For this review, use the dimensioned drawing (mm, ordinates from the lowest corner) and the shaded views. Round coordinates to 2 decimals unless told otherwise and drop trailing zeros. Loops run counter-clockwise (first coordinate to the right, second up) from the corner with the lowest first, then second, coordinate; pieces in that order, holes last. Notation, with made-up numbers: M 62.5,42.25 L 75.5,42.25 A13 cw 75.5,57.25 Z; hole C 10,38.5 d6. An arc over 180 degrees is marked long. Use a Markdown table: item, result. Add a question column.
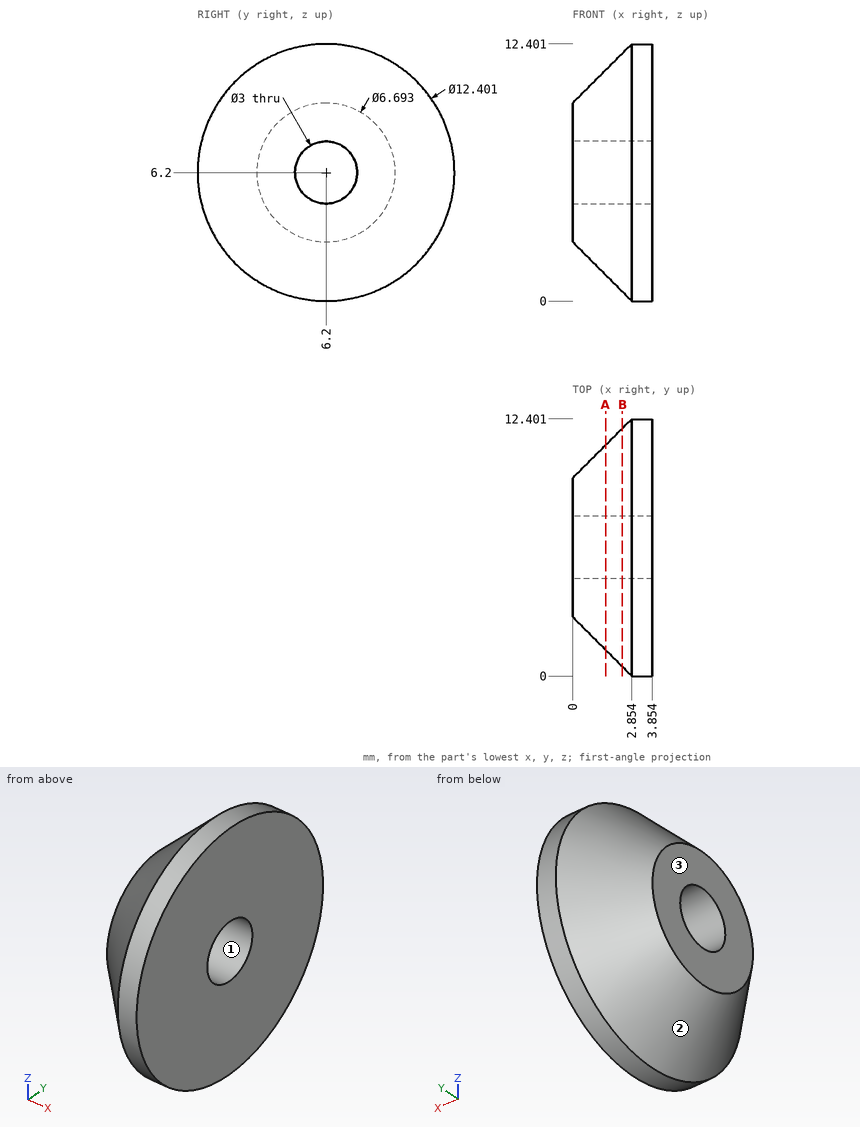
(1) Consider section B-B, the plane x = 2.4. Give the boundary of the cut face in (y, z).
(2) Draft analysis for pull direction Z (two halves, no side actions). For the marked faces 1, 2 and 3, state which applies: released by +Z, released by -Z, zero draft, split by the parting line, or undercut.
(3) To check wall thickness, follow probe 1 along Y at (x, z) = (1.45, 6.5) (1 decimal); probe 2 along Z at (x, y) = (1.7, 6.75) (1 decimal); probe 3 along Y at (x, z) = (3, 5) (1 decimal). State the ranges of each line that lie inside material, in increasing order.
(4) Consider section A-A, the plane x = 1.6. Give the boundary of the cut face in (y, z), then the cut area to 3 significant figures.
(5) Insertion check: pin 1 Ø1 at (x, z) = (1, 7.5) entering from -Y (1 decimal); pin 2 Ø2 at (x, z) = (1, 2) entering from -Y; pin 3 Ø1 at (x, y) = (1, 2.5) entering from +Z (1 decimal). Each pin has a flat end and moves straight along its axis. Give the tip position at first contact, or say it passes through.
Found:
| question | item | result |
|---|---|---|
| 1 | outline | C 6.2,6.2 d11.49; hole C 6.2,6.2 d3 |
| 2 | face 1 | undercut |
| 2 | face 2 | split by the parting line |
| 2 | face 3 | zero draft |
| 3 | probe 1 | y = 1.4 to 4.7, 7.7 to 11 |
| 3 | probe 2 | z = 1.2 to 4.8, 7.6 to 11.2 |
| 3 | probe 3 | y = 0.1 to 5.3, 7.1 to 12.3 |
| 4 | outline | C 6.2,6.2 d9.89; hole C 6.2,6.2 d3 |
| 4 | area | 69.8 mm^2 |
| 5 | pin 1 | stops at y = 1.5 |
| 5 | pin 2 | stops at y = 2.52 |
| 5 | pin 3 | stops at z = 9.5 |
